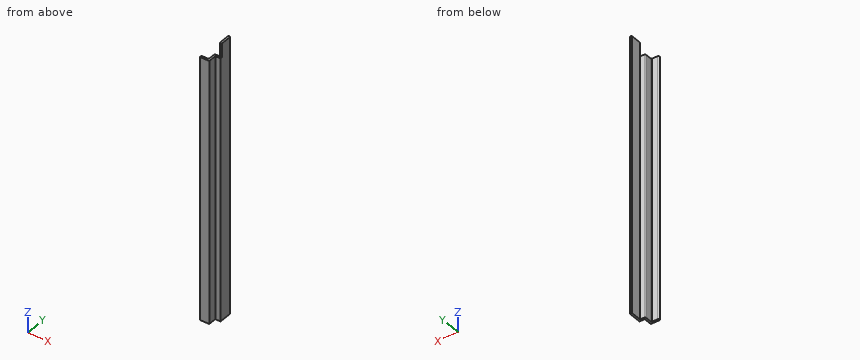
Autodesk Inventor part; units mm, degrees
ref_plane "Work Plane4" through (-4.5, 7.5, 0) normal (-1, 0, 0) x (0, 0, 1)
ref_plane "Work Plane3" through (-4.5, 7.5, 0) normal (-1, 0, 0) x (0, 0, 1)
ref_plane "Work Plane2" through (-4.5, 7.5, 0) normal (-1, 0, 0) x (0, 0, 1)
sketch "Sketch1" plane through (0, 0, 0) normal (0, 0, 1) x (1, 0, 0)
  line L0 (0, 0) -> (-20.5, 0)
  line L1 (-20.5, 0) -> (-20.5, 48)
  line L2 (11.5, 18) -> (0, 18)
  line L3 (0, 18) -> (0, 0)
  line L4 (-20.5, 48) -> (11.5, 48)
  line L5 (11.5, 48) -> (11.5, 18)
  line L6 (-20.5, 0) -> (0, 0)
  line L7 (0, 0) -> (0, 3.5)
  line L8 (-20.5, 3.5) -> (-20.5, 0)
  line L9 (0, 18) -> (11.5, 18)
  line L10 (11.5, 18) -> (11.5, 21.0352)
  line L11 (-20.5, 0) -> (0, 0)
  line L12 (0, 0) -> (0, 4.5)
  line L13 (-20.5, 4.5) -> (-20.5, 0)
  line L14 (-4.5, 22.5) -> (-4.5, 4.5)
  line L15 (-4.5, 4.5) -> (-20.5, 4.5)
  line L16 (-4.5, 22.5) -> (7, 22.5)
  line L17 (7, 22.5) -> (7, 48)
  point P0 (-2.8995, 48)
  dimension "d0" = 20.5
  dimension "d1" = 48
  dimension "d9" = 30
  dimension "d10" = 32
  dimension "d11" = 11.5
  dimension "d16" = 16
  dimension "d23" = 4.5
  dimension "d24" = 4.5
  dimension "d25" = 4.5
extrude "Extrusion2" add sketch "Sketch1" along normal blind 600 contours L0 L1 L15 L14 L16 L17 L4 L5 L2 L3
ref_plane "Work Plane4" through (-4.5, 7.5, 0) normal (-1, 0, 0) x (0, 0, 1)
ref_plane "Work Plane3" through (-4.5, 7.5, 0) normal (-1, 0, 0) x (0, 0, 1)
ref_plane "Work Plane2" through (-4.5, 7.5, 0) normal (-1, 0, 0) x (0, 0, 1)
ref_plane "Work Plane1" through (-4.5, 7.5, 0) normal (-1, 0, 0) x (0, 0, 1)
sketch "Sketch7" plane through (-20.5, 0, 0) normal (-1, 0, 0) x (0, 0, 1)
  line L0 (600, 22.5) -> (600, 4.5)
  line L1 (0, 0) -> (600, 0)
  line L2 (660, 22.5) -> (0, 22.5)
  line L3 (600, 0) -> (570, 0)
  line L4 (570, 0) -> (570, 22.5)
  line L5 (570, 22.5) -> (600, 22.5)
  line L6 (600, 22.5) -> (600, 0)
  point P0 (660, 19.5)
  point P1 (660, 7.5)
  dimension "d71" = 30
extrude "Extrusion4" cut sketch "Sketch7" along normal mid plane 1000
fillet "Fillet4" radius 2 5 edges at (-20.5, 4.5, 285) (-4.5, 22.5, 285) (7, 48, 300) (11.5, 48, 300) (-4.5, 4.5, 285)
properties part number "gancho"
Work out the finished part from the listing and answer in its coordinate system (mm). Round coordinates to 2 decimals unless told otherwise and drop trailing zeros. Write each loop counter-clockwise with the first axis right and the second up, starting at its lowest first coordinate (ties: lowest second). Pieces come first, ordered by that corner, then holes. Notation, with made-up numbers: (59, -14) -> (76, -14) arc R9 cw to (76, -5) -> close; hole circle Ø2 at (-39, 78). An arc over 180 degrees is marked (long way). Write each question's results on one line, items separated by ' | '.
Q1. Flat-ended cylindrical pins translate along their axes: P1, Ø5, axis at x = 9.5, z = 586.5, coming from the -Y side; P2, Ø15.5, axis at y = 11, z = 367.5, coming from the -X side; P3, Ø12, axis at x = -4.5, z = 305.5, coming from the +Y side; P4, Ø5, axis at x = -5.5, y = 25.5, coming from the -Z side. Find the tip coordinate at first contact, or state that the pin passes through.
Data:
P1: y = 22.5 | P2: x = -20.35 | P3: y = 22.5 | P4: through
Q2. Straight lines are drawn through the part: line 1 along Y through (x, z) = (0.5, 30); line 2 along X through (y, z) = (36, 143.5); line 3 along X through (y, z) = (19, 174). For each, find the intervals that lie inside material, in ascending order. Write a range as [from, to].
Data:
line 1: [18, 22.5] | line 2: [7, 11.5] | line 3: [-4.5, 11.5]
Q3. Section A-A, the plane z = 484.5 is taken. Write down the section's boundary in (x, y).
Data:
outline: (-20.5, 0) -> (0, 0) -> (0, 18) -> (11.5, 18) -> (11.5, 46) arc R2 ccw to (9.5, 48) -> (9, 48) arc R2 ccw to (7, 46) -> (7, 22.5) -> (-2.5, 22.5) arc R2 ccw to (-4.5, 20.5) -> (-4.5, 6.5) arc R2 cw to (-6.5, 4.5) -> (-18.5, 4.5) arc R2 ccw to (-20.5, 2.5) -> close
Q4. Section B-B, the plane y = 33.5 is taken. Write down the section's boundary in (x, z), then the cut area to 3 significant figures.
Data:
outline: (7, 0) -> (11.5, 0) -> (11.5, 600) -> (7, 600) -> close | area: 2,700 mm^2
